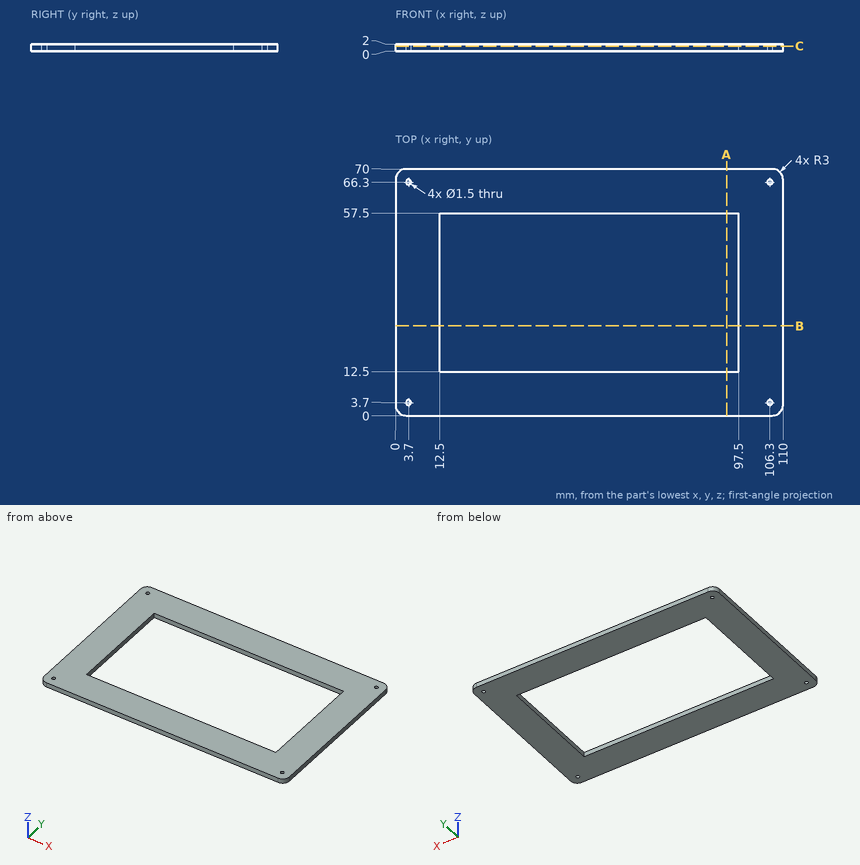
Answer from the drawing. Dimensions are ordinates in mm from the lowest x, y and z of the part. Coordinates: 2 decimals unless noted, no trailing zeros. Order: outer loops, then holes, each group sorted by start corner. A loop starts at its lowest first (then second) coordinate and runs counter-clockwise, first axis right, second up. Notation, with made-up numbers: M 23.25,89 L 53.25,89 A27 ccw 53.25,117 Z; hole C -37.5,-14.75 d3. An arc over 180 degrees is marked long. Put each result on its own line as item: value. Start each with the question number.
Item 1: Section C-C, the plane z = 1.4 is taken. Determine the outline of the cut face in (x, y).
Item 2: Consider probe 1 along X at (y, z) = (66.3, 0.65); probe 2 along Y at (x, z) = (106.3, 1.05); probe 3 along X at (y, z) = (52.5, 1.5). Determine where each line is inside the solid, lowest interval first. Write a range as [from, to].
Item 3: Section A-A, the plane x = 94 is taken. Determine the outline of the cut face in (y, z).
Item 4: Given pin 1 Ø1.2 at (x, y) = (106.3, 3.7) entering from -Z; pin 2 Ø1 at (x, z) = (31.5, 1) entering from -Y, each flat-ended and moving along its own axis, determine where each tip first touches the part or whether it passes through.
Item 5: Section B-B, the plane y = 25.5 is taken. Determine the outline of the cut face in (x, z).
Computed:
1. outline: M 0,3 A3 ccw 3,0 L 107,0 A3 ccw 110,3 L 110,67 A3 ccw 107,70 L 3,70 A3 ccw 0,67 Z; hole C 3.7,3.7 d1.5; hole C 3.7,66.3 d1.5; hole M 12.5,12.5 L 97.5,12.5 L 97.5,57.5 L 12.5,57.5 Z; hole C 106.3,3.7 d1.5; hole C 106.3,66.3 d1.5
2. probe 1: x = [0, 2.95], [4.45, 105.55], [107.05, 110]
2. probe 2: y = [0, 2.95], [4.45, 65.55], [67.05, 70]
2. probe 3: x = [0, 12.5], [97.5, 110]
3. outline: M 0,0 L 12.5,0 L 12.5,2 L 0,2 Z; M 57.5,0 L 70,0 L 70,2 L 57.5,2 Z
4. pin 1: passes through
4. pin 2: stops at y = 0
5. outline: M 0,0 L 12.5,0 L 12.5,2 L 0,2 Z; M 97.5,0 L 110,0 L 110,2 L 97.5,2 Z
